```python
from build123d import *

# Parameters (mm, degrees)
SKETCH2_R           = 45.43
BOSS_EXTRUDE2_DEPTH = 6
SKETCH3_R           = 12
BOSS_EXTRUDE3_DEPTH = 7
SKETCH4_R           = 6
BOSS_EXTRUDE4_DEPTH = 5
SKETCH5_R           = 3
CUT_EXTRUDE1_DEPTH  = 13
SCALE1_SCALE        = 0.15


with BuildPart() as part:
    # Sketch2 → Boss-Extrude2 (new body)
    with BuildSketch(Plane.XY):
        with Locations((-5.265954001, 0)):
            Circle(SKETCH2_R)
    extrude(amount=BOSS_EXTRUDE2_DEPTH)

    # Sketch3 → Boss-Extrude3 (add)
    with BuildSketch(Plane.XY.offset(6)):
        with Locations((-5.265954001, 0)):
            Circle(SKETCH3_R)
    extrude(amount=BOSS_EXTRUDE3_DEPTH)

    # Sketch4 → Boss-Extrude4 (add)
    with BuildSketch(Plane.XY.offset(13)):
        with Locations((-5.265954001, 0)):
            Circle(SKETCH4_R)
    extrude(amount=BOSS_EXTRUDE4_DEPTH)

    # Sketch5 → Cut-Extrude1 (cut)
    with BuildSketch(Plane(origin=(0, 0, 0), x_dir=(-1, 0, 0), z_dir=(0, 0, -1))):
        with Locations((5.265954001, 0)):
            Circle(SKETCH5_R)
    extrude(amount=-CUT_EXTRUDE1_DEPTH, mode=Mode.SUBTRACT)


with BuildPart() as part_1:
    # Scale1: scaled about (-5.265954001, 0, 3.623777836)
    add(part.part.scale(SCALE1_SCALE).moved(Location((-4.476060901, 0, 3.080211161))))


solid = part_1.part
```
Input: part model. Units: mm. Frame: model coordinates. A direction names the side the tool comes from. Give positions to 0.01 mm unless a question says otherwise; leave off trailing zeros. Order: outer loops, then holes, each group sorted by start corner. A loop starts at its lowest first (then second) coordinate and runs counter-clockwise, first axis right, second up.
1. Section C-C on x = -5. Return the cut outline in (y, z).
Derived:
outline: (-6.81, 3.08) - (-0.36, 3.08) - (-0.36, 5.03) - (0.36, 5.03) - (0.36, 3.08) - (6.81, 3.08) - (6.81, 3.98) - (1.78, 3.98) - (1.78, 5.03) - (0.86, 5.03) - (0.86, 5.78) - (-0.86, 5.78) - (-0.86, 5.03) - (-1.78, 5.03) - (-1.78, 3.98) - (-6.81, 3.98) - close
2. Section A-A on y = 0. Return the cut outline in (x, z).
Derived:
outline: (-12.08, 3.08) - (-5.72, 3.08) - (-5.72, 5.03) - (-4.82, 5.03) - (-4.82, 3.08) - (1.55, 3.08) - (1.55, 3.98) - (-3.47, 3.98) - (-3.47, 5.03) - (-4.37, 5.03) - (-4.37, 5.78) - (-6.17, 5.78) - (-6.17, 5.03) - (-7.07, 5.03) - (-7.07, 3.98) - (-12.08, 3.98) - close
3. Reachability of faces 4 (the cylindrical face through (-6.59, 1.22, 4.5)), 5 (the cylindrical face through (-5.695, 0.135, 4.042)), 6 (the flat face through (-4, 0, 3.08)) from +Z, -Z, +X, -X, +Y, -Y: full face, straight path, thin tool, end or side. Return the list, or none.
Derived:
face 4: +Z
face 5: -Z
face 6: -Z, +X, -X, +Y, -Y
4. Section D-D on z = 5.2. Return the cut outline in (x, y), and give its area (3 significant figures).
Derived:
outline: circle Ø1.8 at (-5.27, 0)
area: 2.54 mm2
5. Section B-B on z = 3.4. Return the cut outline in (x, y), and give its area (3 significant figures).
Derived:
outline: circle Ø13.63 at (-5.27, 0); hole circle Ø0.9 at (-5.27, 0)
area: 145 mm2
6. Mould query, pull axis X, two halves, no side actions, for faces 1 (the cylindrical face through (-10.67, -4.15, 3.52)), 2 (the flat face through (-5, 0, 5.03)), 3 (the flat face through (-3.8, -1.4, 3.98)). Classes: released by +X, released by -X, zero draft, split by the parting line, or undercut.
Derived:
face 1: split by the parting line
face 2: undercut
face 3: zero draft
7. Material intervals for L1, parallel to Z at x = -3, y = 0.5; L2, parallel to X at y = -5, z = 3.7; L3, parallel to X at y = 5.5, z = 3.3, sorted ascending.
Derived:
L1: z = 3.08 to 3.98
L2: x = -9.9 to -0.64
L3: x = -9.29 to -1.24
